```python
from build123d import *

# Parameters (mm, degrees)
BOX013_W          = 30.84
BOX013_H          = 6.5
BOX013_DEPTH      = 12.55
BOX014_W          = 6.5
BOX014_H          = 6
BOX014_DEPTH      = 12.55
BOX015_W          = 6.5
BOX015_H          = 6
BOX015_DEPTH      = 12.55
BOX016_W          = 15.8
BOX016_H          = 7
BOX016_DEPTH      = 6.2
BOX017_W          = 23
BOX017_H          = 6
BOX017_DEPTH      = 1.6
BOX018_W          = 19
BOX018_H          = 6
BOX018_DEPTH      = 2
CYLINDER004_R     = 1.42
CYLINDER004_DEPTH = 3
CYLINDER005_R     = 1.42
CYLINDER005_DEPTH = 3
CHAMFER_1_ANGLE   = 10
CHAMFER_1_SIZE    = 4.5
CHAMFER_2_ANGLE   = 10
CHAMFER_2_SIZE    = 4.5
FILLET_R          = 5
FILLET001_R       = 1.5
FILLET002_R       = 5
FILLET003_R       = 1.5
FILLET004_R       = 1.5
FILLET005_R       = 1.5
FILLET006_R       = 0.38
FILLET007_R       = 0.38
BOX031_W          = 1
BOX031_H          = 6
BOX031_DEPTH      = 10
BOX032_W          = 1
BOX032_H          = 6
BOX032_DEPTH      = 10


with BuildPart() as part:
    # Box013 → Box013 (join)
    with BuildSketch(Plane(origin=(-15.42, 19, 0), x_dir=(1, 0, 0), z_dir=(0, 0, 1))):
        with Locations((15.42, 3.25)):
            Rectangle(BOX013_W, BOX013_H)
    extrude(amount=BOX013_DEPTH)

    # Box014 → Box014 (cut)
    with BuildSketch(Plane(origin=(9, 19.5, 0), x_dir=(1, 0, 0), z_dir=(0, 0, 1))):
        with Locations((3.25, 3)):
            Rectangle(BOX014_W, BOX014_H)
    extrude(amount=BOX014_DEPTH, mode=Mode.SUBTRACT)

    # Box015 → Box015 (cut)
    with BuildSketch(Plane(origin=(-15.5, 19.5, 0), x_dir=(1, 0, 0), z_dir=(0, 0, 1))):
        with Locations((3.25, 3)):
            Rectangle(BOX015_W, BOX015_H)
    extrude(amount=BOX015_DEPTH, mode=Mode.SUBTRACT)

    # Box016 → Box016 (cut)
    with BuildSketch(Plane(origin=(-7.9, 19, 3), x_dir=(1, 0, 0), z_dir=(0, 0, 1))):
        with Locations((7.9, 3.5)):
            Rectangle(BOX016_W, BOX016_H)
    extrude(amount=BOX016_DEPTH, mode=Mode.SUBTRACT)

    # Box017 → Box017 (cut)
    with BuildSketch(Plane(origin=(-11.5, 19.5, 0), x_dir=(1, 0, 0), z_dir=(0, 0, 1))):
        with Locations((11.5, 3)):
            Rectangle(BOX017_W, BOX017_H)
    extrude(amount=BOX017_DEPTH, mode=Mode.SUBTRACT)

    # Box018 → Box018 (cut)
    with BuildSketch(Plane(origin=(-9.5, 19.5, 10.55), x_dir=(1, 0, 0), z_dir=(0, 0, 1))):
        with Locations((9.5, 3)):
            Rectangle(BOX018_W, BOX018_H)
    extrude(amount=BOX018_DEPTH, mode=Mode.SUBTRACT)

    # Cylinder004 → Cylinder004 (cut)
    with BuildSketch(Plane(origin=(12.5, 21, 6.3), x_dir=(1, 0, 0), z_dir=(0, -1, 0))):
        Circle(CYLINDER004_R)
    extrude(amount=CYLINDER004_DEPTH, mode=Mode.SUBTRACT)

    # Cylinder005 → Cylinder005 (cut)
    with BuildSketch(Plane(origin=(-12.5, 20, 6.3), x_dir=(1, 0, 0), z_dir=(0, -1, 0))):
        Circle(CYLINDER005_R)
    extrude(amount=CYLINDER005_DEPTH, mode=Mode.SUBTRACT)

    # Chamfer 1
    chamfer_1_edges = [part.edges().sort_by_distance(p)[0] for p in [
        (7.9, 22.25, 3),
    ]]
    chamfer_1_side = part.faces().sort_by_distance((7.9, 22.25, 6.1))[0]
    chamfer(chamfer_1_edges, length=CHAMFER_1_SIZE, angle=CHAMFER_1_ANGLE, reference=chamfer_1_side)

    # Chamfer 2
    chamfer_2_edges = [part.edges().sort_by_distance(p)[0] for p in [
        (-7.9, 22.25, 3),
    ]]
    chamfer_2_side = part.faces().sort_by_distance((-7.9, 22.25, 6.1))[0]
    chamfer(chamfer_2_edges, length=CHAMFER_2_SIZE, angle=CHAMFER_2_ANGLE, reference=chamfer_2_side)

    # Fillet
    fillet_edges = [part.edges().sort_by_distance(p)[0] for p in [
        (7.9, 22.25, 7.5),
    ]]
    fillet(fillet_edges, radius=FILLET_R)

    # Fillet001
    fillet001_edges = [part.edges().sort_by_distance(p)[0] for p in [
        (7.9, 22.25, 9.2),
    ]]
    fillet(fillet001_edges, radius=FILLET001_R)

    # Fillet002
    fillet002_edges = [part.edges().sort_by_distance(p)[0] for p in [
        (-7.9, 22.25, 7.5),
    ]]
    fillet(fillet002_edges, radius=FILLET002_R)

    # Fillet003
    fillet003_edges = [part.edges().sort_by_distance(p)[0] for p in [
        (-7.9, 22.25, 9.2),
    ]]
    fillet(fillet003_edges, radius=FILLET003_R)

    # Fillet004
    fillet004_edges = [part.edges().sort_by_distance(p)[0] for p in [
        (7.106529, 22.25, 3),
    ]]
    fillet(fillet004_edges, radius=FILLET004_R)

    # Fillet005
    fillet005_edges = [part.edges().sort_by_distance(p)[0] for p in [
        (-7.106529, 22.25, 3),
    ]]
    fillet(fillet005_edges, radius=FILLET005_R)

    # Cone → Cone (revolve, cut)
    with BuildSketch(Plane(origin=(12.5, 19.5, 6.3), x_dir=(1, 0, 0), z_dir=(0, 0, -1))):
        Polygon((0, 0), (2.42, 0), (1.32, 0.2), (0, 0.2), align=None)
    revolve(axis=Axis((12.5, 19.5, 6.3), (0, -1, 0)), mode=Mode.SUBTRACT)

    # Fillet006
    fillet006_edges = [part.edges().sort_by_distance(p)[0] for p in [
        (11.08, 19.318182, 6.3),
    ]]
    fillet(fillet006_edges, radius=FILLET006_R)

    # Cone001 → Cone001 (revolve, cut)
    with BuildSketch(Plane(origin=(-12.5, 19.5, 6.3), x_dir=(1, 0, 0), z_dir=(0, 0, -1))):
        Polygon((0, 0), (2.42, 0), (1.32, 0.2), (0, 0.2), align=None)
    revolve(axis=Axis((-12.5, 19.5, 6.3), (0, -1, 0)), mode=Mode.SUBTRACT)

    # Fillet007
    fillet007_edges = [part.edges().sort_by_distance(p)[0] for p in [
        (-13.92, 19.318182, 6.3),
    ]]
    fillet(fillet007_edges, radius=FILLET007_R)

    # Box031 → Box031 (cut)
    with BuildSketch(Plane(origin=(8, 19.5, 0), x_dir=(0.984808, 0, -0.173648), z_dir=(0.173648, 0, 0.984808))):
        with Locations((0.5, 3)):
            Rectangle(BOX031_W, BOX031_H)
    extrude(amount=BOX031_DEPTH, mode=Mode.SUBTRACT)

    # Box032 → Box032 (cut)
    with BuildSketch(Plane(origin=(-9, 19.5, 0), x_dir=(0.984808, 0, 0.173648), z_dir=(-0.173648, 0, 0.984808))):
        with Locations((0.5, 3)):
            Rectangle(BOX032_W, BOX032_H)
    extrude(amount=BOX032_DEPTH, mode=Mode.SUBTRACT)


solid = part.part
```
Check sheet for the modelled part. Datum: model origin and axes. Units: mm. A direction names the side the tool comes from. Round coordinates to 2 decimals unless told otherwise and drop trailing zeros. Order: outer loops, then holes, each group sorted by start corner. A loop starts at its lowest first (then second) coordinate and runs counter-clockwise, first axis right, second up. Notation, with made-up numbers: (-12, 72.25) - (12, 72.25) arc R13 ccw to (12, 82.25) - close; hole circle Ø5 at (74.25, -31.75). An arc over 180 degrees is marked (long way). Write item = value, one per line.
Q1. Draft check along X on faces 6 (the face through (9, 22, 8)), 7 (the face through (-7.57, 22.2, 5.63)), 8 (the face through (0, 19.5, 1)). Enter one of: pulls with the +X half, pulls with the -X half, needs draft (parallel to the pull), parting line crosses it, or undercut.
Computed:
face_6 = pulls with the +X half
face_7 = undercut
face_8 = needs draft
Q2. Section check B-B (z = 1). Record the boundary of the cut face in (x, y), and give its area (3 significant figures).
Computed:
outline = (-15.42, 19) - (15.42, 19) - (15.42, 19.5) - (-15.42, 19.5) - close
area = 15.4 mm^2
Q3. Tool access check on faces 1 (the face through (0, 23, 10.55)), 2 (the face through (-8.63, 22.46, 3.65)), 3 (the face through (-9, 22, 8)), 4 (the face through (8.636, 22.458, 3.607)), 5 (the face through (7.57, 22.2, 5.63)). Record the directions out of +Z, -Z, +X, -X, +Y, -Y that give a thin tool (end or side, any length) a straight path to the whole face; none if there is none.
Computed:
face_1 = +Z, +X, -X, +Y
face_2 = -Z, -X, +Y
face_3 = +Z, -Z, -X, +Y
face_4 = -Z, +X, +Y
face_5 = +Y, -Y
Q4. Thickness scan on line 1 along Z through (x, y) = (5, 20.75); line 2 along Y through (x, z) = (-6, 1.25); line 3 along X through (y, z) = (19.05, 6.3). Record the ranges inside material, lowest first.
Computed:
line_1 = 1.6 to 3, 9.2 to 10.55
line_2 = 19 to 19.5
line_3 = -15.42 to -13.92, -11.08 to -7.69, 7.69 to 11.08, 13.92 to 15.42
Q5. Go/stop test with flat-tipped pins: pin 1 (2 mm diameter, centred on x = 0.5, y = 22, fed in from +Z); pin 2 (1 mm diameter, centred on x = 11.5, z = 5, fed in from +Y); pin 3 (2.5 mm diameter, centred on x = -12.5, z = 6.3, fed in from -Y); pin 4 (1 mm diameter, centred on x = 7.5, z = 7.5, fed in from +Y). Record where each tip stops, or that it passes through.
Computed:
pin_1 = 10.55
pin_2 = 19.45
pin_3 = through
pin_4 = 25.5
Q6. Section check A-A (x = -4). Record the boundary of the cut face in (y, z).
Computed:
outline = (19, 0) - (19.5, 0) - (19.5, 1.6) - (25.5, 1.6) - (25.5, 3) - (19, 3) - close; (19, 9.2) - (25.5, 9.2) - (25.5, 10.55) - (19.5, 10.55) - (19.5, 12.55) - (19, 12.55) - close
Q7. Section check C-C (z = 6.3). State how many separate pieces and enclosed holes the cut face has, and give its area (3 significant figures).
Computed:
separate_pieces = 4
enclosed_holes = 0
area = 20.2 mm^2
